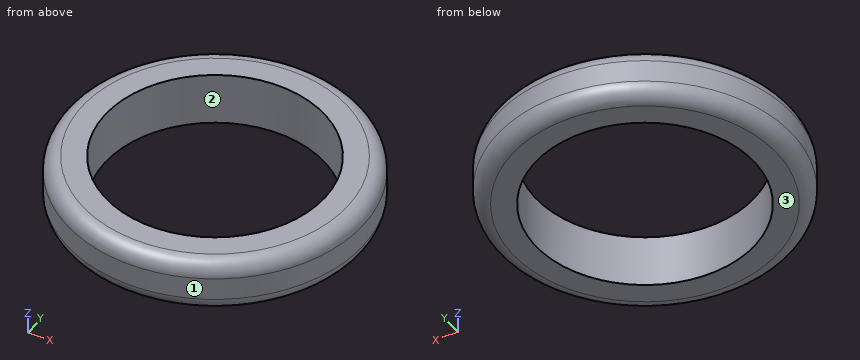
```python
from build123d import *

# Parameters (mm, degrees)
F0_R     = 19.5
F0_R_2   = 14.5
F1_DEPTH = 3.5
F2_R     = 2


with BuildPart() as f1:
    # F0 (on Top) → F1 (new body)
    with BuildSketch(Plane.XY):
        Circle(F0_R)
        Circle(F0_R_2, mode=Mode.SUBTRACT)
    extrude(amount=F1_DEPTH)

    # F2
    f2_edges = [f1.edges().sort_by_distance(p)[0] for p in [
        (-19.5, 0, 3.5),
    ]]
    fillet(f2_edges, radius=F2_R)

    # F3: F1 across plane


with BuildPart() as f1_1:
    add(f1.part)
    add(f1.part.mirror(Plane.XY))


solid = f1_1.part
```
Here's how the part is built. I have some questions about the finished solid (model axes, mm). Face numbers are marked on the shaded views. Round coordinates to 2 decimals unless told otherwise and drop trailing zeros. Write each loop counter-clockwise with the first axis right and the second up, starting at its lowest first coordinate (ties: lowest second). Pieces come first, ordered by that corner, then holes. Notation, with made-up numbers: M 36.25,14.25 L 75.25,14.25 A23 cw 75.25,40.25 Z; hole C -17,71 d3. An arc over 180 degrees is marked long. Answer as CSV lines item,"result". Start each with the question number.
1. I'm going to push flat-ended pins straight in: pin 1 Ø4 at (y, z) = (10, 2.5) entering from +X; pin 2 Ø1.5 at (y, z) = (11, -2.5) entering from +X. Where does each tip first touch, or does it pass through?
2. Suppose I cut it at C-C on z = -0.5. Write out the boundary of the cut face in (x, y), then the cut area to 3 significant figures.
3. Thinking about a two-plate mould opening in Y: for the marked faces 1, 2 and 3, which applies, released by +Y, released by -Y, zero draft, split by the parting line, or undercut?
4. I need wall thicknesses on probe 1 along Y at (x, z) = (0, -1.5); probe 2 along Y at (x, z) = (0, 3); probe 3 along X at (y, z) = (5, 3). Which ranges of each line are inside material? Lowest first, please.
5. Suppose I cut it at A-A on y = 0. Write out the boundary of the cut face in (x, z), then the cut area to 3 significant figures.
Check result:
1,pin 1,"stops at x = 17.7"
1,pin 2,"stops at x = 16.41"
2,outline,"C 0,0 d39; hole C 0,0 d29"
2,area,"534 mm2"
3,face 1,"split by the parting line"
3,face 2,"undercut"
3,face 3,"zero draft"
4,probe 1,"y = -19.5 to -14.5, 14.5 to 19.5"
4,probe 2,"y = -18.82 to -14.5, 14.5 to 18.82"
4,probe 3,"x = -18.15 to -13.61, 13.61 to 18.15"
5,outline,"M -19.5,-1.5 A2 ccw -17.5,-3.5 L -14.5,-3.5 L -14.5,3.5 L -17.5,3.5 A2 ccw -19.5,1.5 Z; M 14.5,-3.5 L 17.5,-3.5 A2 ccw 19.5,-1.5 L 19.5,1.5 A2 ccw 17.5,3.5 L 14.5,3.5 Z"
5,area,"66.6 mm2"
